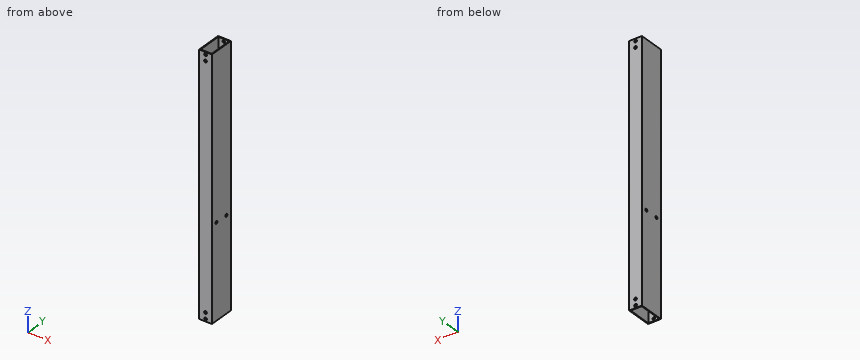
Autodesk Inventor part; units mm, degrees
ref_plane "YZ Plane" through (0, 0, 0) normal (1, 0, 0) x (0, 1, 0)
ref_plane "XZ Plane" through (0, 0, 0) normal (0, 1, 0) x (-1, 0, 0)
ref_plane "XY Plane" through (0, 0, 0) normal (0, 0, 1) x (1, 0, 0)
sketch "スケッチ1" plane through (0, 0, 0) normal (0, 0, 1) x (1, 0, 0)
  line L0 (0, 0) -> (15, 0)
  line L1 (15, 0) -> (15, 30)
  line L2 (15, 30) -> (0, 30)
  line L3 (0, 30) -> (0, 0)
  line L4 (1, 1) -> (14, 1)
  line L5 (14, 1) -> (14, 29)
  line L6 (14, 29) -> (1, 29)
  line L7 (1, 29) -> (1, 1)
  dimension "d0" = 15
  dimension "d1" = 30
  dimension "d2" = 13
  dimension "d3" = 28
  dimension "d4" = 1
  dimension "d5" = 1
extrude "押し出し1" add sketch "スケッチ1" along normal blind 300
sketch "スケッチ2" plane through (0, 30, 0) normal (0, 1, 0) x (1, 0, 0)
  circle A0 centre (7.5, -3) radius 1.6
  line L0 (15, 0) -> (15, -300)
  line L1 (15, 0) -> (0, 0)
  circle A1 centre (7.5, -10) radius 1.6
  line L2 (0, -150) -> (15, -150) construction
  line L3 (15, -300) -> (0, -300)
  circle A2 centre (7.5, -297) radius 1.6
  circle A3 centre (7.5, -290) radius 1.6
  dimension "d8" = 3.2
  dimension "d9" = 7.5
  dimension "d10" = 3
  dimension "d11" = 3.2
  dimension "d12" = 7
  dimension "d13" = 7.5
  dimension "d14" = 150
hole "穴1" at (7.5, 30, 297) at (7.5, 30, 290) at (7.5, 30, 10) at (7.5, 30, 3) direction (0, -1, 0) diameter 3.2 depth 30
sketch "スケッチ3" plane through (15, 0, 0) normal (1, 0, 0) x (0, 0, -1)
  circle A0 centre (-109.5, 23) radius 1.6
  line L0 (0, 0) -> (0, 30)
  line L1 (0, 30) -> (-300, 30)
  circle A1 centre (-109.5, 7) radius 1.6
  line L2 (0, 0) -> (-300, 0)
  dimension "d22" = 3.2
  dimension "d23" = 109.5
  dimension "d24" = 7
  dimension "d25" = 3.2
  dimension "d26" = 16
  dimension "d27" = 7
hole "穴2" at (15, 23, 109.5) at (15, 7, 109.5) direction (-1, 0, 0) diameter 3.2 depth 15
equation "\"BendRadius\" = Thickness"
equation "\"BendReliefWidth\" = Thickness"
equation "\"BendReliefDepth\" = 0.5 * Thickness"
equation "\"CornerReliefSize\" = 4 * Thickness"
equation "\"MinimumRemnant\" = 2 * Thickness"
equation "\"TransitionRadius\" = BendRadius"
equation "\"JacobiRadiusSize\" = BendRadius"
equation "\"GapSize\" = Thickness"
properties part number "nhk48"
Geometry check sheet. Reference: the model listing, model coordinates, mm. Give positions to 0.01 mm unless a question says otherwise; leave off trailing zeros. Loops run counter-clockwise (first coordinate to the right, second up) from the corner with the lowest first, then second, coordinate; pieces in that order, holes last. Notation, with made-up numbers: (-4, -13.5) -> (22, -13.5) arc R16 cw to (22, -1.5) -> close; hole circle Ø4 at (59.25, -32). An arc over 180 degrees is marked (long way). Answer in a Markdown table with one row per item. Add a question column.
1) Gauge pin test, flat end, axial feed: P1, Ø5, axis at x = 7.5, z = 3, coming from the +Y side. Record the tip position at first contact, or that the pin passes through.
2) Cross-section at C-C on z = 105. Record the boundary of the cut face in (x, y), and give its area (3 significant figures).
3) Cross-section at B-B on y = 15.25. Record the boundary of the cut face in (x, z).
4) Cross-section at A-A on x = 3.5. Record the boundary of the cut face in (y, z), and give its area (3 significant figures).
5) Material ranges on probe 1 along Z at (x, y) = (7.5, 0.6); probe 2 along Y at (x, z) = (8, 173.5); probe 3 along X at (y, z) = (9, 83), recorded low to high. Write a range as from..to.
Outcome:
| question | item | result |
|---|---|---|
| 1 | P1 | stops at y = 30 |
| 2 | outline | (0, 0) -> (15, 0) -> (15, 30) -> (0, 30) -> close; hole (1, 1) -> (14, 1) -> (14, 29) -> (1, 29) -> close |
| 2 | area | 86.0 mm^2 |
| 3 | outline | (0, 0) -> (1, 0) -> (1, 300) -> (0, 300) -> close; (14, 0) -> (15, 0) -> (15, 300) -> (14, 300) -> close |
| 4 | outline | (0, 0) -> (1, 0) -> (1, 300) -> (0, 300) -> close; (29, 0) -> (30, 0) -> (30, 300) -> (29, 300) -> close |
| 4 | area | 600 mm^2 |
| 5 | probe 1 | z = 0..1.4, 4.6..8.4, 11.6..288.4, 291.6..295.4, 298.6..300 |
| 5 | probe 2 | y = 0..1, 29..30 |
| 5 | probe 3 | x = 0..1, 14..15 |
